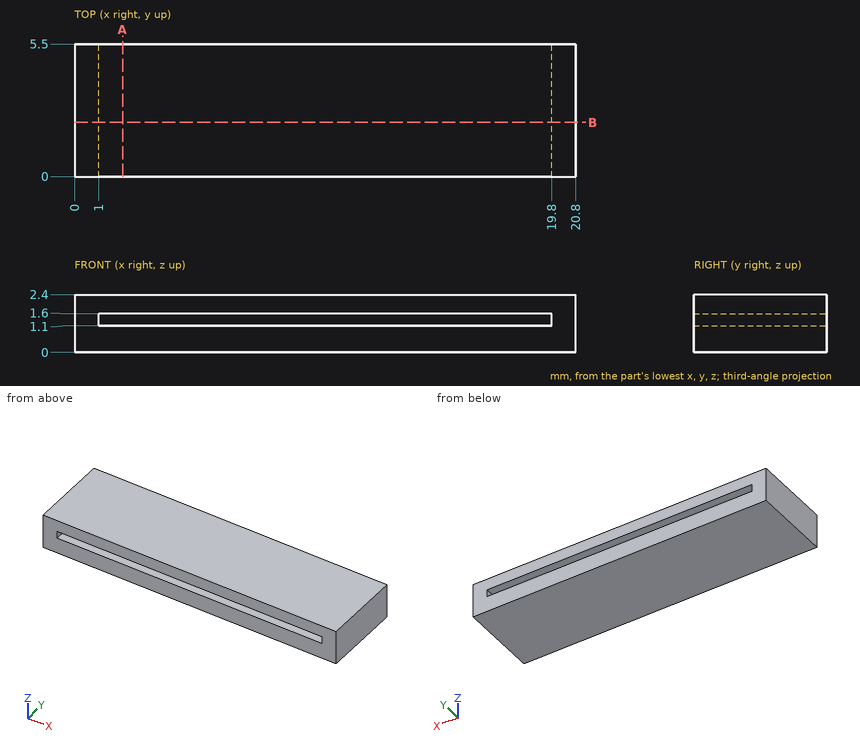
Design review of the part shown in the three views and the two pictorial views. Dimensions are in mm from the part's minimum x, y and z. Coordinates: 2 decimals unless noted, no trailing zeros. Loops run counter-clockwise (first coordinate to the right, second up) from the corner with the lowest first, then second, coordinate; pieces in that order, holes last.
(1) Wall thickness on L1, parallel to Z at x = 16, y = 2.85; L2, parallel to X at y = 0.7, z = 1.4: over which ranges is each line inside the solid? List them lowest first.
Determined:
L1: z = 0 to 1.1, 1.6 to 2.4
L2: x = 0 to 1, 19.8 to 20.8
(2) Consider section B-B, the plane y = 2.25. Give the boundary of the cut face in (x, z).
Determined:
outline: (0, 0) - (20.8, 0) - (20.8, 2.4) - (0, 2.4) - close; hole (1, 1.1) - (19.8, 1.1) - (19.8, 1.6) - (1, 1.6) - close
(3) Insertion check: P1, Ø1.5, axis at x = 9.5, y = 4, coming from the -Z side. The pin has a flat end and moves straight along its axis. Give the tip position at first contact, or say it passes through.
Determined:
P1: stops at z = 0
(4) Consider section A-A, the plane x = 2. Give the boundary of the cut face in (y, z).
Determined:
outline: (0, 0) - (5.5, 0) - (5.5, 1.1) - (0, 1.1) - close; (0, 1.6) - (5.5, 1.6) - (5.5, 2.4) - (0, 2.4) - close
